Work out the finished part from the listing and answer in its coordinate system (mm). Coordinates: 2 decimals unless noted, no trailing zeros. Loops run counter-clockwise (first coordinate to the right, second up) from the corner with the lowest first, then second, coordinate; pieces in that order, holes last. Notation, with made-up numbers: (16.25, -4.5) -> (37.25, -4.5) arc R12 ccw to (37.25, 14.5) -> close; hole circle Ø6 at (31, 78.5). An arc over 180 degrees is marked (long way). One line per question, with ' | ' between items.
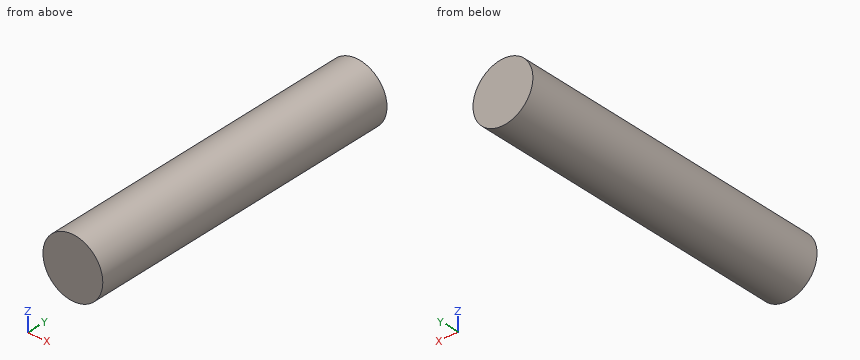
```python
from build123d import *

# Parameters (mm, degrees)
F0_R      = 19.05
F0_R_2    = 15.875
F1_DEPTH  = 203.2
F1_FACE_R = 19.05
F2_DEPTH  = 25.4
F2_FACE_R = 19.05
F3_DEPTH  = 25.4


with BuildPart() as f1:
    # F0 (on Front) → F1 (new body)
    with BuildSketch(Plane.XZ):
        Circle(F0_R)
        Circle(F0_R_2, mode=Mode.SUBTRACT)
        Circle(F0_R_2)
    extrude(amount=F1_DEPTH)

    # F1_face (on face) → F2 (cut)
    with BuildSketch(Plane(origin=(0, 0, 0), x_dir=(1, 0, 0), z_dir=(0, 1, 0))):
        Circle(F1_FACE_R)
    extrude(amount=-F2_DEPTH, mode=Mode.SUBTRACT)

    # F2_face (on face) → F3 (join)
    with BuildSketch(Plane(origin=(0, -25.4, 0), x_dir=(1, 0, 0), z_dir=(0, 1, 0))):
        Circle(F2_FACE_R)
    extrude(amount=F3_DEPTH)


solid = f1.part
```
1) Flat-ended cylindrical pins translate along their axes: pin 1 (5 mm diameter, centred on y = -123, z = 1, fed in from +X); pin 2 (5 mm diameter, centred on x = 13.5, y = -147.5, fed in from +Z); pin 3 (5 mm diameter, centred on x = -9, y = -52.5, fed in from -Z); pin 4 (2 mm diameter, centred on x = -7.5, y = -127.5, fed in from +Z). Find the tip coordinate at first contact, or state that the pin passes through.
Check values:
pin 1: stops at x = 19.05 | pin 2: stops at z = 15.55 | pin 3: stops at z = -17.91 | pin 4: stops at z = 17.91
2) Find section C-C (z = 4). Write down the section's boundary in (x, y).
Check values:
outline: (-18.63, -203.2) -> (18.63, -203.2) -> (18.63, 0) -> (-18.63, 0) -> close
3) Find section B-B (x = -5). Write down the section's boundary in (y, z).
Check values:
outline: (-203.2, -18.38) -> (0, -18.38) -> (0, 18.38) -> (-203.2, 18.38) -> close
4) Find the intervals of material crossed by line 1 along Z through (x, y) = (9, -50); line 2 along X through (y, z) = (-165.5, 12.5); line 3 along X through (y, z) = (-123, 14), in increasing order.
Check values:
line 1: z = -16.79 to 16.79 | line 2: x = -14.38 to 14.38 | line 3: x = -12.92 to 12.92
5) Find section A-A (y = -135). Write down the section's boundary in (x, z), plus the area to 3 significant figures.
Check values:
outline: circle Ø38.1 at (0, 0) | area: 1,140 mm^2
